Input: part model. Units: mm. Frame: model coordinates. A direction names the side the tool comes from. Coordinates: 2 decimals unless noted, no trailing zeros. Order: outer loops, then holes, each group sorted by start corner. A loop starts at its lowest first (then second) coordinate and runs counter-clockwise, first axis right, second up. Notation, with made-up numbers: (-32.5, 88) - (13.5, 88) arc R27 cw to (13.5, 125) - close; hole circle Ø7 at (47, 14). An arc over 180 degrees is marked (long way). One line per question, with ' | ' between items. Start each with the question number.
```python
from build123d import *

# Parameters (mm, degrees)
BOSS_EXTRUDE1_DEPTH = 6.35
CAVITY1_START       = -6.35
CAVITY1_OUTLINE_R   = 12.7
CAVITY1_DEPTH       = 12.7
MOVE_FACE_SLOT_BY   = 0.762
MOVE_FACE_SLOT_2_BY = 0.762
MOVE_FACE_SLOT_3_BY = 0.762
MOVE_FACE_SLOT_4_BY = 0.762
FILLET1_R           = 3.175
MOVE_FACE_HOLE_BY   = 0.635


# Read off the part's stored shape, not the designer's step: Cavity1
with BuildPart() as part:
    # Sketch1 → Boss-Extrude1 (new, symmetric)
    with BuildSketch(Plane.XY):
        Polygon((-215.9, 0), (215.9, 0), (215.9, 25.4), (241.3, 25.4), (241.3, 101.6), (-241.3, 101.6), (-241.3, 25.4), (-215.9, 25.4), align=None)
    extrude(amount=BOSS_EXTRUDE1_DEPTH, both=True)

    # Cavity1 outline → Cavity1 (cut)
    with BuildSketch(Plane.XY.offset(CAVITY1_START)):
        with Locations((50.8, 51.5)):
            Circle(CAVITY1_OUTLINE_R)
    extrude(amount=CAVITY1_DEPTH, mode=Mode.SUBTRACT)

    # Move Face slot: a face moved inward by 0.762
    extrude(part.faces().sort_by_distance((-228.6, 25.4, 0))[0], amount=MOVE_FACE_SLOT_BY, dir=(0, 1, 0), mode=Mode.SUBTRACT)

    # Move Face slot 2: a face moved inward by 0.762
    extrude(part.faces().sort_by_distance((-215.9, 12.7, 0))[0], amount=MOVE_FACE_SLOT_2_BY, dir=(1, 0, 0), mode=Mode.SUBTRACT)

    # Move Face slot 3: a face moved inward by 0.762
    extrude(part.faces().sort_by_distance((215.9, 12.7, 0))[0], amount=MOVE_FACE_SLOT_3_BY, dir=(-1, 0, 0), mode=Mode.SUBTRACT)

    # Move Face slot 4: a face moved inward by 0.762
    extrude(part.faces().sort_by_distance((228.6, 25.4, 0))[0], amount=MOVE_FACE_SLOT_4_BY, dir=(0, 1, 0), mode=Mode.SUBTRACT)

    # Fillet1
    fillet1_edges = [part.edges().sort_by_distance(p)[0] for p in [
        (215.138, 0, 0),
        (215.138, 26.162, 0),
        (241.3, 26.162, 0),
        (241.3, 101.6, 0),
        (-241.3, 101.6, 0),
        (-241.3, 26.162, 0),
        (-215.138, 26.162, 0),
        (-215.138, 0, 0),
    ]]
    fillet(fillet1_edges, radius=FILLET1_R)

    # Move Face hole: a curved face moved inward by 0.635
    add(Solid.thicken(part.faces().sort_by_distance((38.1, 51.5, 0))[0], -MOVE_FACE_HOLE_BY), mode=Mode.SUBTRACT)


solid = part.part
```
(1) Section C-C (y = 51.5). Output: boundary loops of the cut face in (x, z) (3 decimals), then the cut area to 3 significant figures.
(2) Material intervals for line 1 along Y through (x, z) = (50.8, 1) (3 decimals); line 2 along X through (y, z) = (52, -2.75); line 3 along Y through (x, z) = (-218.5, -4), sorted ascending. Write a range as from..to.
(3) Section B-B (z = 0.5). Output: boundary loops of the cut face in (x, y) (3 decimals).
(4) Draft query along Y for faces 1 (the face through (3, 101.6, 0)), 2 (the face through (-3, 52, 6.35)), 3 (the face through (56.95, 39.67, -0.09)). Return one class per face: +Y half, -Y half, draft (parallel to the pull), parting line (faces both ways), or undercut.
(5) Section A-A (x = 50.8). Output: boundary loops of the cut face in (y, z) (3 decimals), then the cut area to 3 significant figures.
(6) Pin query (flat end, axial travel): pin 1 (6.5 mm diameter, centred on x = 228, z = -3, fed in from -Y); pin 2 (1 mm diameter, centred on y = 11, z = -4.5, fed in from +X). Return the tip coordinate at first contact, or that it passes through.
(7) Reachability of faces 4 (the face through (-3, 0, 0)), 5 (the face through (228, 26.162, 0)), 6 (the face through (-228, 26.162, 0)) from +Z, -Z, +X, -X, +Y, -Y: full face, straight path, thin tool, end or side. Return the list, or none.
Worked answers:
1) outline: (-241.3, -6.35) - (37.465, -6.35) - (37.465, 6.35) - (-241.3, 6.35) - close; (64.135, -6.35) - (241.3, -6.35) - (241.3, 6.35) - (64.135, 6.35) - close | area: 5,790 mm²
2) line 1: y = 0..38.165, 64.835..101.6 | line 2: x = -241.3..37.47, 64.13..241.3 | line 3: y = 26.16..101.6
3) outline: (-241.3, 29.337) arc R3.175 ccw to (-238.125, 26.162) - (-218.313, 26.162) arc R3.175 cw to (-215.138, 22.987) - (-215.138, 3.175) arc R3.175 ccw to (-211.963, 0) - (211.963, 0) arc R3.175 ccw to (215.138, 3.175) - (215.138, 22.987) arc R3.175 cw to (218.313, 26.162) - (238.125, 26.162) arc R3.175 ccw to (241.3, 29.337) - (241.3, 98.425) arc R3.175 ccw to (238.125, 101.6) - (-238.125, 101.6) arc R3.175 ccw to (-241.3, 98.425) - close; hole circle Ø26.67 at (50.8, 51.5)
4) face 1: +Y half | face 2: draft | face 3: undercut
5) outline: (0, -6.35) - (38.165, -6.35) - (38.165, 6.35) - (0, 6.35) - close; (64.835, -6.35) - (101.6, -6.35) - (101.6, 6.35) - (64.835, 6.35) - close | area: 952 mm²
6) pin 1: stops at y = 26.16 | pin 2: stops at x = 215.14
7) face 4: +Z, -Z, +X, -X, -Y | face 5: +Z, -Z, +X, -Y | face 6: +Z, -Z, -X, -Y
